Check sheet for the modelled part. Datum: model origin and axes. Units: mm. Face numbers are marked on the shaded views. Coordinates: 2 decimals unless noted, no trailing zeros. Order: outer loops, then holes, each group sorted by start corner. A loop starts at its lowest first (then second) coordinate and runs counter-clockwise, first axis right, second up.
1. Gauge pin test, flat ends, axial feed: pin 1 Ø2 at (y, z) = (-656.5, 32.5) entering from +X; pin 2 Ø2 at (x, z) = (123.5, 47.5) entering from +Y; pin 3 Ø1 at (x, z) = (-261, 71) entering from +Y. Record the tip position at first contact, or that the pin passes through.
2. Cross-section at D-D (x = 179). Enter the section's corners in (y, z), then the cut area to 3 significant figures.
3. Cross-section at B-B (y = -482.5). Enter the section's corners in (x, z), then the cut area to 3 significant figures.
4. Draft check along X on the marked faces 1 and 2. Enter one of: released by +X, released by -X, zero draft, split by the parting line, or undercut.
5. Cross-section at C-C (y = 700.5). Enter the section's corners in (x, z), then the cut area to 3 significant figures.
6. Thickness scan on line 1 (X direction, y = -684, z = 22.5); line 2 (X direction, y = -660, z = 64); line 3 (Y direction, x = 16, z = 91). Record the ranges inside material, lowest first.
7. Cross-section at A-A (y = 457). Enter the section's corners in (x, z).
```python
from build123d import *

# Parameters (mm, degrees)
F0_W      = 762
F0_H      = 1828.8
F1_DEPTH  = 114.3
F2_W      = 35.56
F2_H      = 114.3
F3_DEPTH  = 114.3
F4_W      = 152.4
F4_H      = 1143
F5_DEPTH  = 76.2
F6_W      = 35.56
F6_H      = 304.8
F7_DEPTH  = 114.3
F9_DEPTH  = 35.56
F11_DEPTH = 35.56
F12_R     = 8.73125
F13_DEPTH = 114.3


with BuildPart() as f1:
    # F0 (on Top) → F1 (new body)
    with BuildSketch(Plane.XY):
        Rectangle(F0_W, F0_H)
    extrude(amount=F1_DEPTH)

    # F2 (on face) → F3 (cut, through all)
    with BuildSketch(Plane.XY.offset(114.3)):
        with Locations((-292.1, 476.25)):
            Rectangle(F2_W, F2_H)
        with Locations((292.1, 476.25)):
            Rectangle(F2_W, F2_H)
        with Locations((-292.1, -704.85)):
            Rectangle(F2_W, F2_H)
        with Locations((292.1, -704.85)):
            Rectangle(F2_W, F2_H)
        with Locations((-363.22, 476.25)):
            Rectangle(F2_W, F2_H)
        with Locations((-363.22, -704.85)):
            Rectangle(F2_W, F2_H)
        with Locations((363.22, 476.25)):
            Rectangle(F2_W, F2_H)
        with Locations((363.22, -704.85)):
            Rectangle(F2_W, F2_H)
    extrude(amount=-F3_DEPTH, mode=Mode.SUBTRACT)

    # F4 (on face) → F5 (cut)
    with BuildSketch(Plane.XY.offset(114.3)):
        with Locations((0, -38.1)):
            Rectangle(F4_W, F4_H)
    extrude(amount=-F5_DEPTH, mode=Mode.SUBTRACT)

    # F6 (on face) → F7 (cut, through all)
    with BuildSketch(Plane.XY.offset(114.3)):
        with Locations((-256.54, 762)):
            Rectangle(F6_W, F6_H)
    extrude(amount=-F7_DEPTH, mode=Mode.SUBTRACT)

    # F8 (on face) → F9 (join)
    with BuildSketch(Plane(origin=(-381, 0, 0), x_dir=(0, -1, 0), z_dir=(-1, 0, 0))):
        Polygon((-914.4, 25.4), (-914.4, 88.9), (-949.96, 95.170187), (-949.96, 19.129813), align=None)
    extrude(amount=-F9_DEPTH)

    # F10 (on face) → F11 (join)
    with BuildSketch(Plane.YZ.offset(381)):
        Polygon((949.96, 95.170187), (914.4, 88.9), (914.4, 25.4), (949.96, 19.129813), align=None)
    extrude(amount=-F11_DEPTH)

    # F12 (on face) → F13 (cut, through all)
    with BuildSketch(Plane.XY.offset(114.3)):
        with Locations((-256.54, 558.8)):
            Circle(F12_R)
        with Locations((-256.54, 406.4)):
            Circle(F12_R)
        with Locations((-256.54, 254)):
            Circle(F12_R)
        with Locations((-256.54, 101.6)):
            Circle(F12_R)
        with Locations((-256.54, -50.8)):
            Circle(F12_R)
        with Locations((-256.54, -203.2)):
            Circle(F12_R)
        with Locations((-256.54, -355.6)):
            Circle(F12_R)
        with Locations((-256.54, -508)):
            Circle(F12_R)
        with Locations((-256.54, -660.4)):
            Circle(F12_R)
        with Locations((-256.54, -812.8)):
            Circle(F12_R)
    extrude(amount=-F13_DEPTH, mode=Mode.SUBTRACT)


solid = f1.part
```
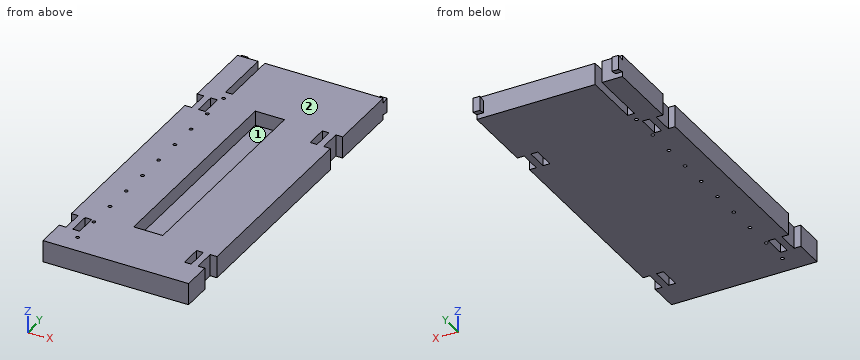
Data:
1. pin 1: stops at x = 345.44
1. pin 2: stops at y = 914.4
1. pin 3: stops at y = 609.6
2. outline: (-914.4, 0) - (914.4, 0) - (914.4, 114.3) - (-914.4, 114.3) - close
2. area: 209,000 mm2
3. outline: (-381, 0) - (381, 0) - (381, 114.3) - (76.2, 114.3) - (76.2, 38.1) - (-76.2, 38.1) - (-76.2, 114.3) - (-381, 114.3) - close
3. area: 75,500 mm2
4. face 1: undercut
4. face 2: zero draft
5. outline: (-381, 0) - (-274.32, 0) - (-274.32, 114.3) - (-381, 114.3) - close; (-238.76, 0) - (381, 0) - (381, 114.3) - (-238.76, 114.3) - close
5. area: 83,000 mm2
6. line 1: x = -345.44 to -309.88, -274.32 to 274.32, 309.88 to 345.44
6. line 2: x = -345.44 to -309.88, -274.32 to -265.26, -247.82 to 274.32, 309.88 to 345.44
6. line 3: y = -914.4 to -609.6, 533.4 to 914.4
7. outline: (-345.44, 0) - (-309.88, 0) - (-309.88, 114.3) - (-345.44, 114.3) - close; (-274.32, 0) - (274.32, 0) - (274.32, 114.3) - (76.2, 114.3) - (76.2, 38.1) - (-76.2, 38.1) - (-76.2, 114.3) - (-274.32, 114.3) - close; (309.88, 0) - (345.44, 0) - (345.44, 114.3) - (309.88, 114.3) - close
